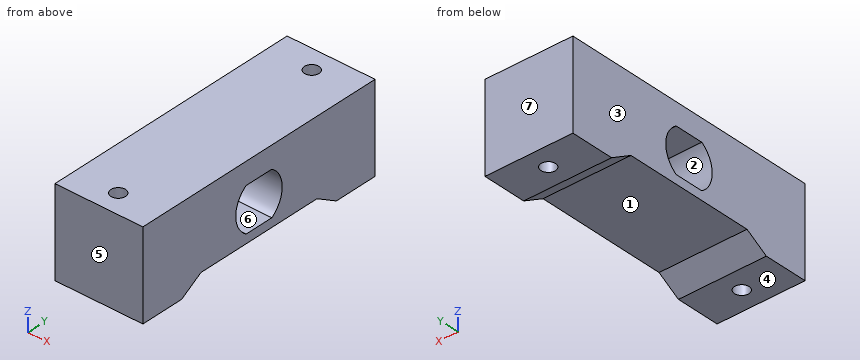
Autodesk Fusion 360 part; units mm, degrees
sketch "Sketch1" plane through (0, 0, 0) normal (0, 0, 1) x (1, 0, 0)
  line L0 (0, 0) -> (20, 0)
  line L1 (20, 0) -> (20, 60)
  line L2 (20, 60) -> (0, 60)
  line L3 (0, 60) -> (0, 0)
extrude "Extrude1" add sketch "Sketch1" along normal blind 30
extrude "Extrude2" cut 1 faces at (6.6667, 40, 30) along direction (0, 0, -1) blind 10
sketch "Sketch2" plane through (20, 0, 0) normal (1, 0, 0) x (0, 1, 0)
  line L0 (60, 20) -> (0, 20)
  line L1 (0, 20) -> (0, 0)
  line L2 (0, 0) -> (60, 0)
  line L3 (60, 0) -> (60, 20)
  line L4 (36, 5) -> (24, 5)
  line L5 (24, 5) -> (24, 15)
  line L6 (24, 15) -> (36, 15)
  line L7 (36, 15) -> (36, 5)
  line L8 (36, 5) -> (24, 15) construction
  line L9 (24, 5) -> (36, 15) construction
  circle A0 centre (30, 10) radius 6
  point P0 (30, 10)
extrude "Extrude3" cut sketch "Sketch2" against normal blind 29 contours L4 L6 A0
sketch "Sketch3" plane through (0, 0, 0) normal (0, 0, -1) x (1, 0, 0)
  line L0 (0, 0) -> (0, -60)
  line L1 (0, -60) -> (20, -60)
  line L2 (20, -60) -> (20, 0)
  line L3 (20, 0) -> (0, 0)
  circle A0 centre (10, -5) radius 1.65
  circle A1 centre (10, -55) radius 1.65
  dimension "d7" = 3.3
  dimension "d8" = 3.3
extrude "Extrude4" cut sketch "Sketch3" against normal blind 45 contours A0 | A1
sketch "Sketch4" plane through (20, 0, 0) normal (1, 0, 0) x (0, 1, 0)
  line L0 (33.3166, 5) -> (26.6834, 5)
  arc A0 (26.6834, 15) -> (26.6834, 5) centre (30, 10) ccw
  line L1 (26.6834, 15) -> (33.3166, 15)
  arc A1 (33.3166, 5) -> (33.3166, 15) centre (30, 10) ccw
  line L2 (60, 20) -> (0, 20)
  line L3 (0, 20) -> (0, 0)
  line L4 (0, 0) -> (60, 0)
  line L5 (60, 0) -> (60, 20)
  line L6 (10, 0) -> (15, 3)
  line L7 (15, 3) -> (45, 3)
  line L8 (45, 3) -> (50, 0)
extrude "Extrude5" cut sketch "Sketch4" against normal blind 43 contours L4 L6 L7 L8
The listing builds one solid part. Answer for the finished solid, in the listing's coordinates (mm). Face numbers are marked on the shaded views. A direction names the side the tool comes from. Coordinates: 2 decimals unless noted, no trailing zeros. Write each loop counter-clockwise with the first axis right and the second up, starting at its lowest first coordinate (ties: lowest second). Pieces come first, ordered by that corner, then holes. Notation, with made-up numbers: (24, -19) - (58, -19) arc R26 cw to (58, 16) - close; hole circle Ø11 at (-18, 75.5). An arc over 180 degrees is marked (long way). Return JSON: item names as keys, results as strings.
1. The part is cut by section A-A on x = 10. Determine the outline of the cut face in (y, z), then the cut area to 3 significant figures.
Final values:
{"outline": "(0, 0) - (3.35, 0) - (3.35, 20) - (0, 20) - close; (6.65, 0) - (10, 0) - (15, 3) - (45, 3) - (50, 0) - (53.35, 0) - (53.35, 20) - (6.65, 20) - close; (56.65, 0) - (60, 0) - (60, 20) - (56.65, 20) - close; hole (26.68, 5) - (33.32, 5) arc R6 ccw to (33.32, 15) - (26.68, 15) arc R6 ccw to start", "area": "859 mm^2"}
2. The part is cut by section D-D on x = 18.25. Determine the outline of the cut face in (y, z), then the cut area to 3 significant figures.
Final values:
{"outline": "(0, 0) - (10, 0) - (15, 3) - (45, 3) - (50, 0) - (60, 0) - (60, 20) - (0, 20) - close; hole (26.68, 5) - (33.32, 5) arc R6 ccw to (33.32, 15) - (26.68, 15) arc R6 ccw to start", "area": "991 mm^2"}
3. The part is cut by section C-C on z = 1.5. Determine the outline of the cut face in (x, y), then the cut area to 3 significant figures.
Final values:
{"outline": "(0, 0) - (20, 0) - (20, 12.5) - (0, 12.5) - close; (0, 47.5) - (20, 47.5) - (20, 60) - (0, 60) - close; hole circle Ø3.3 at (10, 5); hole circle Ø3.3 at (10, 55)", "area": "483 mm^2"}
4. Consider line 1 along Y through (x, z) = (10.75, 16.5); line 2 along Y through (x, z) = (10, 13.75); line 3 along Y through (x, z) = (10, 13). Determine where each line is inside the solid, lowest interval first.
Final values:
{"line 1": "0 to 3.53, 6.47 to 53.53, 56.47 to 60", "line 2": "0 to 3.35, 6.65 to 25.32, 34.68 to 53.35, 56.65 to 60", "line 3": "0 to 3.35, 6.65 to 24.8, 35.2 to 53.35, 56.65 to 60"}
5. The part is cut by section B-B on y = 27.5. Determine the outline of the cut face in (x, z).
Final values:
{"outline": "(0, 3) - (20, 3) - (20, 5) - (0, 5) - close; (0, 15) - (20, 15) - (20, 20) - (0, 20) - close"}
6. For a pull along Y with two mould halves and no side action, classify the marked faces 4, 5, 6 and 7 as +Y half, -Y half, draft (parallel to the pull), parting line (faces both ways), or undercut.
Final values:
{"face 4": "draft", "face 5": "-Y half", "face 6": "undercut", "face 7": "+Y half"}
7. This flat-tipped pin is pushed along its axis until it touches: pin 1 Ø5.5 at (x, y) = (7.5, 29.5) entering from -Z. Where does it stop, or does it pass through?
Final values:
{"pin 1": "z = 3"}
8. Which of the six approach directions +Z, -Z, +X, -X, +Y, -Y give full straight-line access (tool end or side, diameter ignored) to the marked faces 1, 2 and 3?
Final values:
{"face 1": "-Z, +X, -X", "face 2": "+X, -X", "face 3": "+Z, -Z, -X, +Y, -Y"}
